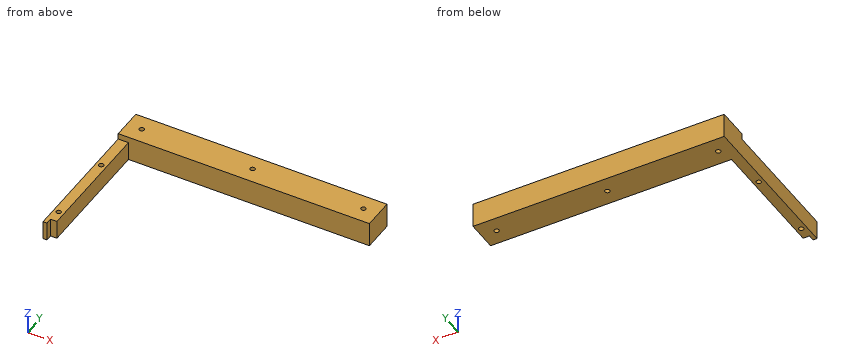
from build123d import *

# Parameters (mm, degrees)
SZKIC1_W                    = 48.766356044
SZKIC1_H                    = 9.435580599
DODANIE_WYCI_GNI_CIE1_DEPTH = 10
SZKIC2_W                    = 48.766356044
SZKIC2_H                    = 9.435580599
DODANIE_WYCI_GNI_CIE2_DEPTH = 2
SZKIC5_W                    = 12
SZKIC5_H                    = 9.435580599
DODANIE_WYCI_GNI_CIE3_DEPTH = 73.233643957
SZKIC6_W                    = 122
SZKIC6_H                    = 12
DODANIE_WYCI_GNI_CIE4_DEPTH = 5.564419
SZKIC7_W                    = 3.404574644
SZKIC7_H                    = 12
DODANIE_WYCI_GNI_CIE5_DEPTH = 64
SZKIC8_W                    = 12
SZKIC8_H                    = 3.048992282
WYTNIJ_WYCI_GNI_CIE1_DEPTH  = 1.5
SZKIC9_R                    = 1.15
WYTNIJ_WYCI_GNI_CIE2_DEPTH  = 130.048184814
SZKIC10_W                   = 12
SZKIC10_H                   = 60.951007718
DODANIE_WYCI_GNI_CIE6_DEPTH = 1.6
SZKIC11_R                   = 1.15
WYTNIJ_WYCI_GNI_CIE3_DEPTH  = 130.048184814
WYTNIJ_WYCI_GNI_CIE4_REACH  = 136.855
SZKIC12_W                   = 2.9
SZKIC12_H                   = 64


with BuildPart() as part:
    # Szkic1 → Dodanie-wyciągnięcie1 (new body)
    with BuildSketch(Plane.XY):
        with Locations((-17.932561551, 12.523716149)):
            Rectangle(SZKIC1_W, SZKIC1_H)
    extrude(amount=DODANIE_WYCI_GNI_CIE1_DEPTH)

    # Szkic2 → Dodanie-wyciągnięcie2 (add)
    with BuildSketch(Plane.XY.offset(10)):
        with Locations((-17.932561551, 12.523716149)):
            Rectangle(SZKIC2_W, SZKIC2_H)
    extrude(amount=DODANIE_WYCI_GNI_CIE2_DEPTH)

    # Szkic5 → Dodanie-wyciągnięcie3 (add)
    with BuildSketch(Plane.ZY.offset(42.315739573)):
        with Locations((6, 12.523716149)):
            Rectangle(SZKIC5_W, SZKIC5_H)
    extrude(amount=DODANIE_WYCI_GNI_CIE3_DEPTH)

    # Szkic6 → Dodanie-wyciągnięcie4 (add)
    with BuildSketch(Plane(origin=(0, 17.241506448, 0), x_dir=(1, 0, 0), z_dir=(0, 1, 0))):
        with Locations((-54.549383529, -6)):
            Rectangle(SZKIC6_W, SZKIC6_H)
    extrude(amount=DODANIE_WYCI_GNI_CIE4_DEPTH)

    # Szkic7 → Dodanie-wyciągnięcie5 (add)
    with BuildSketch(Plane.XZ.offset(-7.805925849)):
        with Locations((-113.847096207, 6)):
            Rectangle(SZKIC7_W, SZKIC7_H)
    extrude(amount=DODANIE_WYCI_GNI_CIE5_DEPTH)

    # Szkic8 → Wytnij-wyciągnięcie1 (cut)
    with BuildSketch(Plane(origin=(-112.144808885, 0, 0), x_dir=(0, 0, -1), z_dir=(1, 0, 0))):
        with Locations((-6, -54.66957801)):
            Rectangle(SZKIC8_W, SZKIC8_H)
    extrude(amount=-WYTNIJ_WYCI_GNI_CIE1_DEPTH, mode=Mode.SUBTRACT)

    # Szkic9 → Wytnij-wyciągnięcie2 (cut, through all)
    with BuildSketch(Plane.XY.offset(12)):
        with Locations((-54.549383529, 15.305925849)):
            Circle(SZKIC9_R)
        with Locations((-108.373957188, 15.305925849)):
            Circle(SZKIC9_R)
        with Locations(Location((-0.724809871, 15.305925849, 0), (0, 0, 180))):
            Circle(SZKIC9_R)
    extrude(amount=-WYTNIJ_WYCI_GNI_CIE2_DEPTH, mode=Mode.SUBTRACT)

    # Szkic10 → Dodanie-wyciągnięcie6 (add)
    with BuildSketch(Plane(origin=(-112.144808885, 0, 0), x_dir=(0, 0, -1), z_dir=(1, 0, 0))):
        with Locations((-6, -22.66957801)):
            Rectangle(SZKIC10_W, SZKIC10_H)
    extrude(amount=DODANIE_WYCI_GNI_CIE6_DEPTH)

    # Szkic11 → Wytnij-wyciągnięcie3 (cut, through all)
    with BuildSketch(Plane.XY.offset(12)):
        with Locations((-113.047096207, -47.199394186)):
            Circle(SZKIC11_R)
        with Locations((-113.047096207, -10.996775314)):
            Circle(SZKIC11_R)
    extrude(amount=-WYTNIJ_WYCI_GNI_CIE3_DEPTH, mode=Mode.SUBTRACT)

    # Wytnij-wyciągnięcie4: up to this face of the body (flat: up to its plane)
    wytnij_wyci_gni_cie4_end = Plane(part.part.faces().sort_by_distance((-110.544808885, -22.66957801, 6))[0])
    # Szkic12 → Wytnij-wyciągnięcie4 (cut, up to the picked face)
    with BuildSketch(Plane.ZY.offset(115.549383529), mode=Mode.PRIVATE) as wytnij_wyci_gni_cie4_sk1:
        with Locations((10.55, -24.194074151)):
            Rectangle(SZKIC12_W, SZKIC12_H)
    wytnij_wyci_gni_cie4_tool1 = split(extrude(wytnij_wyci_gni_cie4_sk1.sketch, amount=-WYTNIJ_WYCI_GNI_CIE4_REACH, mode=Mode.PRIVATE), bisect_by=wytnij_wyci_gni_cie4_end, keep=Keep.BOTH, mode=Mode.PRIVATE)
    add(wytnij_wyci_gni_cie4_tool1.solids().sort_by(Axis((-115.549384, -24.194074, 10.55), (1, 0, 0)))[0], mode=Mode.SUBTRACT)


solid = part.part
Verification items for the finished model (mm, model axes). Give positions to 0.01 mm unless a question says otherwise; leave off trailing zeros. Loops run counter-clockwise (first coordinate to the right, second up) from the corner with the lowest first, then second, coordinate; pieces in that order, holes last.
1) Sectioned sample at B-B, the plane y = 6. Enter the section's corners in (x, z), then the cut area to 3 significant figures.
2) Sectioned sample at C-C, the plane z = 10.75. Enter the section's corners in (x, y), then the cut area to 3 significant figures.
3) Depth check by flat-ended pin: pin 1 Ø1 at (x, y) = (-103, 8.5) entering from -Z; pin 2 Ø4 at (x, y) = (-112, -13) entering from +Z; pin 3 Ø5 at (x, z) = (-12.5, 7.5) entering from -Y; pin 4 Ø1.5 at (y, z) = (-55, 3) entering from +X. Enter the tip coordinate at first touch or a pass-through.
4) Sectioned sample at D-D, the plane x = -10.5. Enter the section's corners in (y, z).
5) Sectioned sample at A-A, the plane z = 5.25. Enter the section's corners in (x, y).
6) Thickness scan on line 1 along X through (y, z) = (-47, 6.5); line 2 along X through (y, z) = (-21, 8); line 3 along Y through (x, z) = (-25, 11). Record the ranges inside material, lowest first.
Answers:
1. outline: (-115.55, 0) - (-110.54, 0) - (-110.54, 9.1) - (-115.55, 9.1) - close
1. area: 45.5 mm2
2. outline: (-115.55, 7.81) - (6.45, 7.81) - (6.45, 22.81) - (-115.55, 22.81) - close; hole circle Ø2.3 at (-108.37, 15.31); hole circle Ø2.3 at (-54.55, 15.31); hole circle Ø2.3 at (-0.72, 15.31)
2. area: 1,820 mm2
3. pin 1: stops at z = 0
3. pin 2: stops at z = 9.1
3. pin 3: stops at y = 7.81
3. pin 4: stops at x = -113.64
4. outline: (7.81, 0) - (22.81, 0) - (22.81, 12) - (7.81, 12) - close
5. outline: (-115.55, -56.19) - (-113.64, -56.19) - (-113.64, -53.15) - (-110.54, -53.15) - (-110.54, 7.81) - (6.45, 7.81) - (6.45, 22.81) - (-115.55, 22.81) - close; hole circle Ø2.3 at (-113.05, -47.2); hole circle Ø2.3 at (-113.05, -11); hole circle Ø2.3 at (-108.37, 15.31); hole circle Ø2.3 at (-54.55, 15.31); hole circle Ø2.3 at (-0.72, 15.31)
6. line 1: x = -115.55 to -114.18, -111.91 to -110.54
6. line 2: x = -115.55 to -110.54
6. line 3: y = 7.81 to 22.81
